CAD build for the part. Positions are in the model's coordinates, mm. A direction names the side the tool comes from. Coordinates: 2 decimals unless noted, no trailing zeros. Write each loop counter-clockwise with the first axis right and the second up, starting at its lowest first coordinate (ties: lowest second). Pieces come first, ordered by that corner, then holes. Notation, with made-up numbers: (26, 38) -> (33, 38) arc R20 cw to (33, 70) -> close; hole circle Ø11 at (-21.5, 68). An arc over 180 degrees is marked (long way). Answer as CSV lines item,"result".
Autodesk Inventor part; units mm, degrees
ref_plane "YZ Plane" through (0, 0, 0) normal (1, 0, 0) x (0, 1, 0)
ref_plane "XZ Plane" through (0, 0, 0) normal (0, 1, 0) x (-1, 0, 0)
ref_plane "XY Plane" through (0, 0, 0) normal (0, 0, 1) x (1, 0, 0)
sketch "草图1" plane through (0, 0, 0) normal (0, 0, 1) x (1, 0, 0)
  circle A0 centre (0, 0) radius 100
  line L0 (-25, -96.8246) -> (25, -96.8246)
  line L1 (25, -96.8246) -> (25, -118)
  line L2 (25, -118) -> (-25, -118)
  line L3 (-25, -118) -> (-25, -96.8246)
  arc A1 (-33, 97.5705) -> (-28, -99.1211) centre (0, 0) ccw
  line L4 (-28, -118) -> (-28, -99.1211)
  line L5 (-28, -118) -> (-25, -118)
  line L6 (-30, 95.3939) -> (-30, 127.5705)
  line L7 (-30, 127.5705) -> (-33, 127.5705)
  line L8 (-33, 127.5705) -> (-33, 97.5705)
  line L9 (0, -100) -> (25, -100)
  dimension "d0" = 200
  dimension "d2" = 50
  dimension "d3" = 33
  dimension "d4" = 3
  dimension "d5" = 3
  dimension "d6" = 3
  dimension "d7" = 30
  dimension "d10" = 18
extrude "拉伸1" add sketch "草图1" against normal blind 398 contours A0 L3 L5 L4 A1 L8 L7 L6
sketch "草图2" plane through (-28, -118, 0) normal (-1, 0, 0) x (0, 0, 1)
  circle A0 centre (-53, 10) radius 2.5
  circle A1 centre (-105, 10) radius 2.5
  line L0 (0, 18.8789) -> (0, 0)
  line L1 (0, 0) -> (-398, 0)
  point P0 (0, 118)
  dimension "d11" = 5
  dimension "d12" = 5
  dimension "d13" = 53
  dimension "d14" = 105
  dimension "d15" = 10
  dimension "d16" = 10
extrude "拉伸2" cut sketch "草图2" against normal blind 3
pattern_linear "矩形阵列1" count 3 spacing 120 along (0, 0, -1) of "拉伸2"
sketch "草图3" plane through (-33, 97.5705, 0) normal (-1, 0, 0) x (0, 0, 1)
  circle A0 centre (-8, 15) radius 2.5
  circle A1 centre (-30, 15) radius 2.5
  line L0 (0, 30) -> (0, 0)
  line L1 (0, 30) -> (-398, 30)
  point P0 (0, -97.5705)
  dimension "d22" = 5
  dimension "d23" = 5
  dimension "d24" = 8
  dimension "d25" = 30
  dimension "d26" = 15
  dimension "d27" = 15
extrude "拉伸3" cut sketch "草图3" against normal blind 3
pattern_linear "矩形阵列2" count 4 spacing 120 along (0, 0, -1) of "拉伸3"
properties part number "装填斗罩"
Item 1: Two-plate mould, pull along Y, no slides. Class faces 4 (the cylindrical face through (-102.997, -0.786, -196.214)), 5 (the flat face through (-30, 111, -196)), 6 (the cylindrical face through (-99.997, -0.792, -196.214)): pulls with the +Y half, pulls with the -Y half, needs draft (parallel to the pull), parting line crosses it, or undercut.
Answer below:
face 4,"parting line crosses it"
face 5,"needs draft"
face 6,"undercut"
Item 2: Saw through at D-D on x = -63. Give the cut face in (y, z), and give its area (3 significant figures).
Answer below:
outline,"(-81.49, -398) -> (-77.66, -398) -> (-77.66, 0) -> (-81.49, 0) -> close; (77.66, -398) -> (81.49, -398) -> (81.49, 0) -> (77.66, 0) -> close"
area,"3,050 mm2"
Item 3: Wall check: line 1 (Y direction, x = -43.5, z = -127.5); line 2 (Y direction, x = -27.25, z = -53); line 3 (X direction, y = -3, z = -229). Give the ranges that are in metal, low to high. Write a range as from..to.
Answer below:
line 1,"y = -93.36..-90.04, 90.04..93.36"
line 2,"y = -118..-110.5, -105.5..-96.22"
line 3,"x = -102.96..-99.95"
Item 4: Saw through at B-B on z = -329.5. Give the cut face in (x, y), and give its area (3 significant figures).
Answer below:
outline,"(-33, 97.57) arc R103 ccw to (-28, -99.12) -> (-28, -118) -> (-25, -118) -> (-25, -96.82) arc R100 cw to (-30, 95.39) -> (-30, 127.57) -> (-33, 127.57) -> close"
area,"933 mm2"
Item 5: Saw through at C-C on y = 31.5. Give the cut face in (x, z).
Answer below:
outline,"(-98.07, -398) -> (-94.91, -398) -> (-94.91, 0) -> (-98.07, 0) -> close"
Item 6: 3-axis set-ups, long thin cutter, end or side, ignore diameter. For faces 1 (the flat face through (-102, 5, 0)), 2 (the flat face through (-33, 113, -196)), 3 (the flat face through (-28, -109, -196)): which of +Z, -Z, +X, -X, +Y, -Y reach the whole face in a straight line?
Answer below:
face 1,"+Z, +X, -X, +Y, -Y"
face 2,"+Z, -Z, -X, +Y"
face 3,"+Z, -Z, -X, -Y"
Item 7: Saw through at A-A on x = -42. Give the cut face in (y, z).
Answer below:
outline,"(-94.05, -398) -> (-90.75, -398) -> (-90.75, 0) -> (-94.05, 0) -> close; (90.75, -398) -> (94.05, -398) -> (94.05, 0) -> (90.75, 0) -> close"
Item 8: Flat gauge pins, fed straight in: pin 1 (3 mm diameter, centred on y = -108, z = -105, fed in from +X); pin 2 (24 mm diameter, centred on y = 114.5, z = -217, fed in from -X); pin 3 (6 mm diameter, centred on y = 112.57, z = -128, fed in from +X); pin 4 (4 mm diameter, centred on y = -93, z = -69.5, fed in from -X). Where does each tip first touch, or does it go through?
Answer below:
pin 1,"passes through"
pin 2,"stops at x = -33"
pin 3,"stops at x = -30"
pin 4,"stops at x = -48.25"
